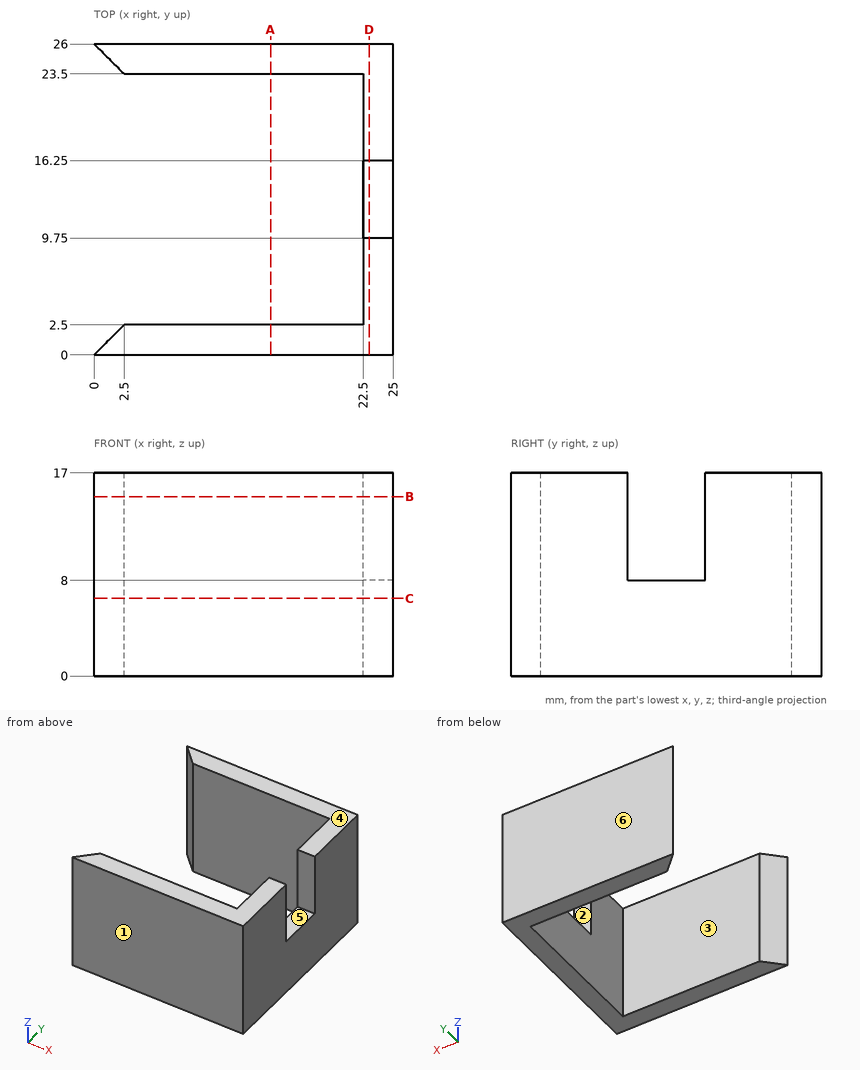
Print and shaded views of the part. All mm, measured from the part's lowest x, y and z. A direction names the side the tool comes from. Give positions to 0.01 mm unless a question says otherwise; leave off trailing zeros. Loops run counter-clockwise (first coordinate to the right, second up) from the corner with the lowest first, then second, coordinate; pieces in that order, holes last. Notation, with made-up numbers: (-33, 70) -> (-12, 70) arc R6 cw to (-12, 76) -> close; hole circle Ø9 at (58.25, -21). An arc over 180 degrees is marked (long way). Use CSV: the item, a comma, the result in double quotes. Start each with the question number.
1) Mould opens along Y. For the marked faces 4, 5 and 6 say: released by +Y, released by -Y, zero draft, split by the parting line, or undercut.
2) Slice it at B-B on z = 15. Give the cut face in (x, y).
3) Tool access for the marked faces 1, 2 and 3: list every direction of +Z, -Z, +X, -X, +Y, -Y with a clear straight run to the whole face (end or side of a thin tool).
4) Slice it at A-A on x = 14.75. Give the cut face in (y, z), plus the area to 3 significant figures.
5) Slice it at C-C on z = 6.5. Give the cut face in (x, y), plus the area to 3 significant figures.
6) Wall check: line 1 (Y direction, x = 16.5, z = 10.5); line 2 (X direction, y = 18, z = 2.25); line 3 (X direction, y = 2, z = 3). Give the ranges that are in metal, low to high.
7) Flat gauge pins, fed straight in: pin 1 Ø5 at (y, z) = (21.5, 15) entering from -X; pin 2 Ø0.8 at (x, y) = (24, 13.5) entering from +Z; pin 3 Ø4 at (y, z) = (3, 9.5) entering from -X. Where does each tip first touch, or does it go through?
8) Slice it at D-D on x = 23. Give the cut face in (y, z), plus the area to 4 significant figures.
Computed values:
1,face 4,"zero draft"
1,face 5,"undercut"
1,face 6,"released by +Y"
2,outline,"(0, 0) -> (25, 0) -> (25, 9.75) -> (22.5, 9.75) -> (22.5, 2.5) -> (2.5, 2.5) -> close; (0, 26) -> (2.5, 23.5) -> (22.5, 23.5) -> (22.5, 16.25) -> (25, 16.25) -> (25, 26) -> close"
3,face 1,"+Z, -Z, +X, -X, -Y"
3,face 2,"+Z, +X, -X"
3,face 3,"+Z, -Z, -X"
4,outline,"(0, 0) -> (2.5, 0) -> (2.5, 17) -> (0, 17) -> close; (23.5, 0) -> (26, 0) -> (26, 17) -> (23.5, 17) -> close"
4,area,"85.0 mm^2"
5,outline,"(0, 0) -> (25, 0) -> (25, 26) -> (0, 26) -> (2.5, 23.5) -> (22.5, 23.5) -> (22.5, 2.5) -> (2.5, 2.5) -> close"
5,area,"171 mm^2"
6,line 1,"y = 0 to 2.5, 23.5 to 26"
6,line 2,"x = 22.5 to 25"
6,line 3,"x = 2 to 25"
7,pin 1,"stops at x = 2"
7,pin 2,"stops at z = 8"
7,pin 3,"stops at x = 1"
8,outline,"(0, 0) -> (26, 0) -> (26, 17) -> (16.25, 17) -> (16.25, 8) -> (9.75, 8) -> (9.75, 17) -> (0, 17) -> close"
8,area,"383.5 mm^2"
